```python
from build123d import *

# Parameters (mm, degrees)
SKETCH_1_W          = 2.91
SKETCH_1_H          = 12.7
EXTRUDE_1_DEPTH     = 3
EXTRUDE_2_DEPTH     = 3
CUT_EXTRUDE_3_DEPTH = 3
SKETCH_3_W          = 1.93
SKETCH_3_H          = 2.895
CUT_EXTRUDE_1_DEPTH = 3


with BuildPart() as part:
    # 스케치1 → 보스-돌출1 (new body)
    with BuildSketch(Plane(origin=(0, 0, 0), x_dir=(1, 0, 0), z_dir=(0, 1, 0))):
        Polygon((-17, -33.75), (-17, 33.75), (-4.66, 33.75), (-1.75, 33.75), (1.75, 33.75), (4.66, 33.75), (17, 33.75), (17, -33.75), (4.66, -33.75), (4.66, -19.81), (1.75, -19.81), (1.75, -33.75), (-1.75, -33.75), (-1.75, -19.81), (-4.66, -19.81), (-4.66, -33.75), align=None)
        with Locations((-3.205, 11.24)):
            Rectangle(SKETCH_1_W, SKETCH_1_H, mode=Mode.SUBTRACT)
        with Locations((-3.205, -7.46)):
            Rectangle(SKETCH_1_W, SKETCH_1_H, mode=Mode.SUBTRACT)
        with Locations((3.205, 11.24)):
            Rectangle(SKETCH_1_W, SKETCH_1_H, mode=Mode.SUBTRACT)
        with Locations((3.205, -7.46)):
            Rectangle(SKETCH_1_W, SKETCH_1_H, mode=Mode.SUBTRACT)
    extrude(amount=EXTRUDE_1_DEPTH)

    # 스케치2 → 보스-돌출2 (add)
    with BuildSketch(Plane(origin=(0, 3, 0), x_dir=(1, 0, 0), z_dir=(0, 1, 0))):
        with BuildLine():
            Line((-17, -33.75), (-17, 33.75))
            ThreePointArc((-17, 33.75), (-37.789714209, 0), (-17, -33.75))
        make_face()
        with BuildLine():
            ThreePointArc((-17, -33.75), (0, -37.789714209), (17, -33.75))
            Line((17, -33.75), (4.66, -33.75))
            Line((4.66, -33.75), (1.75, -33.75))
            Line((1.75, -33.75), (-1.75, -33.75))
            Line((-1.75, -33.75), (-4.66, -33.75))
            Line((-4.66, -33.75), (-17, -33.75))
        make_face()
        with BuildLine():
            ThreePointArc((37.789714209, 0), (32.175205062, 19.819653862), (17, 33.75))
            Line((17, 33.75), (17, -33.75))
            ThreePointArc((17, -33.75), (32.175205062, -19.819653862), (37.789714209, 0))
        make_face()
        with BuildLine():
            Line((-17, 33.75), (17, 33.75))
            ThreePointArc((17, 33.75), (0, 37.789714209), (-17, 33.75))
        make_face()
    extrude(amount=-EXTRUDE_2_DEPTH)

    # 스케치5 → 컷-돌출3 (cut)
    with BuildSketch(Plane(origin=(0, 3, 0), x_dir=(1, 0, 0), z_dir=(0, 1, 0))):
        with BuildLine():
            Line((-34.476203601, -4.66), (-31.537469067, -4.66))
            Line((-31.537469067, -4.66), (-31.537469067, 14.687146066))
            ThreePointArc((-31.537469067, 14.687146066), (-34.395192397, 5.224457362), (-34.476203601, -4.66))
        make_face()
        with BuildLine():
            Line((-24.537469067, 24.662457836), (-24.537469067, -4.66))
            Line((-24.537469067, -4.66), (-21.598734534, -4.66))
            Line((-21.598734534, -4.66), (-21.598734534, 27.273043125))
            ThreePointArc((-21.598734534, 27.273043125), (-23.10500183, 26.009288825), (-24.537469067, 24.662457836))
        make_face()
        with BuildLine():
            Line((-14.598734534, 31.578492123), (-14.598734534, -4.66))
            Line((-14.598734534, -4.66), (-11.66, -4.66))
            Line((-11.66, -4.66), (-11.66, 32.777562672))
            ThreePointArc((-11.66, 32.777562672), (-13.143048633, 32.211558288), (-14.598734534, 31.578492123))
        make_face()
        with BuildLine():
            Line((31.578492123, 14.598734534), (11.66, 14.598734534))
            Line((11.66, 14.598734534), (11.66, 11.66))
            Line((11.66, 11.66), (32.777562672, 11.66))
            ThreePointArc((32.777562672, 11.66), (32.211558288, 13.143048633), (31.578492123, 14.598734534))
        make_face()
        with BuildLine():
            Line((24.662457836, 24.537469067), (11.66, 24.537469067))
            Line((11.66, 24.537469067), (11.66, 21.598734534))
            Line((11.66, 21.598734534), (27.273043125, 21.598734534))
            ThreePointArc((27.273043125, 21.598734534), (26.009288825, 23.10500183), (24.662457836, 24.537469067))
        make_face()
        with BuildLine():
            Line((11.66, 31.537469067), (14.687146066, 31.537469067))
            ThreePointArc((14.687146066, 31.537469067), (13.188156979, 32.193116194), (11.66, 32.777562672))
            Line((11.66, 32.777562672), (11.66, 31.537469067))
        make_face()
        with BuildLine():
            Line((14.598734534, -31.578492123), (14.598734534, 4.66))
            Line((14.598734534, 4.66), (11.66, 4.66))
            Line((11.66, 4.66), (11.66, -32.777562672))
            ThreePointArc((11.66, -32.777562672), (13.143048633, -32.211558288), (14.598734534, -31.578492123))
        make_face()
        with BuildLine():
            Line((24.537469067, -24.662457836), (24.537469067, 4.66))
            Line((24.537469067, 4.66), (21.598734534, 4.66))
            Line((21.598734534, 4.66), (21.598734534, -27.273043125))
            ThreePointArc((21.598734534, -27.273043125), (23.10500183, -26.009288825), (24.537469067, -24.662457836))
        make_face()
        with BuildLine():
            Line((31.537469067, 4.66), (31.537469067, -14.687146066))
            ThreePointArc((31.537469067, -14.687146066), (34.395192397, -5.224457362), (34.476203601, 4.66))
            Line((34.476203601, 4.66), (31.537469067, 4.66))
        make_face()
        with BuildLine():
            Line((-31.578492123, -14.598734534), (-11.66, -14.598734534))
            Line((-11.66, -14.598734534), (-11.66, -11.66))
            Line((-11.66, -11.66), (-32.777562672, -11.66))
            ThreePointArc((-32.777562672, -11.66), (-32.211558288, -13.143048633), (-31.578492123, -14.598734534))
        make_face()
        with BuildLine():
            Line((-24.662457836, -24.537469067), (-11.66, -24.537469067))
            Line((-11.66, -24.537469067), (-11.66, -21.598734534))
            Line((-11.66, -21.598734534), (-27.273043125, -21.598734534))
            ThreePointArc((-27.273043125, -21.598734534), (-26.009288825, -23.10500183), (-24.662457836, -24.537469067))
        make_face()
        with BuildLine():
            Line((-11.66, -31.537469067), (-14.687146066, -31.537469067))
            ThreePointArc((-14.687146066, -31.537469067), (-13.188156979, -32.193116194), (-11.66, -32.777562672))
            Line((-11.66, -32.777562672), (-11.66, -31.537469067))
        make_face()
    extrude(amount=-CUT_EXTRUDE_3_DEPTH, mode=Mode.SUBTRACT)

    # 스케치3 → 컷-돌출1 (cut)
    with BuildSketch(Plane(origin=(0, 3, 0), x_dir=(1, 0, 0), z_dir=(0, 1, 0))):
        Polygon((-13.921720976, -29.640380671), (-16.485116171, -28.295007088), (-15.588200449, -26.586076958), (-13.024805254, -27.931450541), align=None)
        Polygon((-29.640380671, 13.921720976), (-28.295007088, 16.485116171), (-26.586076958, 15.588200449), (-27.931450541, 13.024805254), align=None)
        Polygon((13.921720976, 29.640380671), (16.485116171, 28.295007088), (15.588200449, 26.586076958), (13.024805254, 27.931450541), align=None)
        Polygon((26.876754365, 18.708462151), (28.424032932, 16.261636853), (26.792816067, 15.230117809), (25.2455375, 17.676943106), align=None)
        Polygon((29.640380671, -13.921720976), (28.295007088, -16.485116171), (26.586076958, -15.588200449), (27.931450541, -13.024805254), align=None)
        Polygon((-28.294726577, -6.082986865), (-27.545445441, -8.879342132), (-25.681208596, -8.379821375), (-26.430489732, -5.583466108), align=None)
        Polygon((-27.545445441, 8.879342132), (-28.294726577, 6.082986865), (-26.430489732, 5.583466108), (-25.681208596, 8.379821375), align=None)
        Polygon((27.545445441, -8.879342132), (28.294726577, -6.082986865), (26.430489732, -5.583466108), (25.681208596, -8.379821375), align=None)
        Polygon((-18.947986862, -16.900912731), (-16.900912731, -18.947986862), (-15.536196643, -17.583270774), (-17.583270774, -15.536196643), align=None)
        Polygon((-16.900912731, 18.947986862), (-18.947986862, 16.900912731), (-17.583270774, 15.536196643), (-15.536196643, 17.583270774), align=None)
        with BuildLine():
            Line((15.862041837, -7.0175654), (18.772041837, -7.0175654))
            Line((18.772041837, -7.0175654), (18.772041837, -4.1605654))
            Line((18.772041837, -4.1605654), (19.614041677, -4.1605654))
            ThreePointArc((19.614041677, -4.1605654), (19.916683492, -4.035207055), (20.042041837, -3.73256524))
            Line((20.042041837, -3.73256524), (20.042041837, -2.30256556))
            ThreePointArc((20.042041837, -2.30256556), (19.916683492, -1.999923745), (19.614041677, -1.8745654))
            Line((19.614041677, -1.8745654), (18.772041837, -1.8745654))
            Line((18.772041837, -1.8745654), (18.772041837, 0.9824346))
            Line((18.772041837, 0.9824346), (15.862041837, 0.9824346))
            Line((15.862041837, 0.9824346), (15.862041837, -7.0175654))
        make_face()
        Polygon((18.708462151, -26.876754365), (16.261636853, -28.424032932), (15.230117809, -26.792816067), (17.676943106, -25.2455375), align=None)
        Polygon((16.900912731, -18.947986862), (18.947986862, -16.900912731), (17.583270774, -15.536196643), (15.536196643, -17.583270774), align=None)
        Polygon((-10.527707159, 15.339523687), (-8.020563615, 16.787023687), (-7.055563615, 15.115594658), (-9.562707159, 13.668094658), align=None)
        with Locations((-17.583270774, 0)):
            Rectangle(SKETCH_3_W, SKETCH_3_H)
        Polygon((8.020563615, 16.787023687), (10.527707159, 15.339523687), (9.562707159, 13.668094658), (7.055563615, 15.115594658), align=None)
        Polygon((10.527707159, -15.339523687), (8.020563615, -16.787023687), (7.055563615, -15.115594658), (9.562707159, -13.668094658), align=None)
        Polygon((-8.020563615, -16.787023687), (-10.527707159, -15.339523687), (-9.562707159, -13.668094658), (-7.055563615, -15.115594658), align=None)
    extrude(amount=-CUT_EXTRUDE_1_DEPTH, mode=Mode.SUBTRACT)


solid = part.part
```
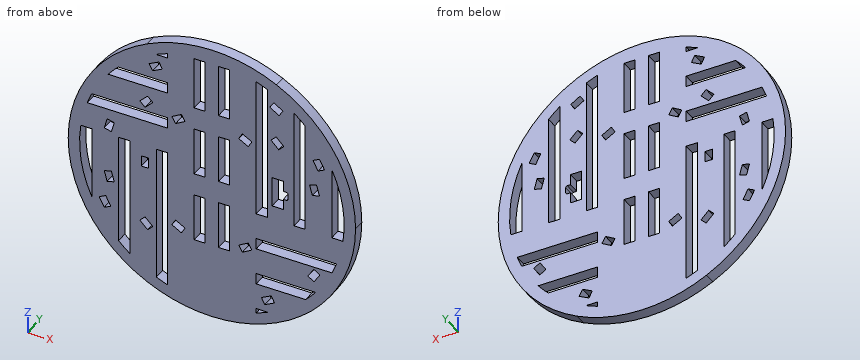
Read the model definition and answer for the solid it produces. Units are mm, in the model's axes. Give positions to 0.01 mm unless a question says otherwise; leave off trailing zeros. Loops run counter-clockwise (first coordinate to the right, second up) from the corner with the lowest first, then second, coordinate; pieces in that order, holes last.
Item 1: The part is cut by section B-B (x = 30.5). Write down the section's boundary in (y, z), and give its area (3 significant figures).
Item 2: Each of these flat-tipped pins is pushed along its axis until it touches: pin 1 Ø0.9 at (x, y) = (17.5, 1.5) entering from -Z; pin 2 Ø1.5 at (x, y) = (2.5, 2) entering from +Z; pin 3 Ø1.5 at (x, y) = (-6.5, 2) entering from -Z. Where does it stop, or does it pass through?
Item 3: Find the intervals of material crossed by line 1 along Z through (x, y) = (-19, 2.1); line 2 along X through (y, z) = (0.55, -24.5); line 3 along X through (y, z) = (1.1, 22), in increasing order.
Item 4: The part is cut by section A-A (z = -3.5). Write down the section's boundary in (x, y).
Item 5: The part is cut by section C-C (y = 1.45). Give the number of separate pieces and of enclosed holes in the cut face, and give its area (3 significant figures).
Taken from the geometry:
1. outline: (0, -22.31) - (3, -22.31) - (3, -14.6) - (0, -14.6) - close; (0, -11.66) - (3, -11.66) - (3, 22.31) - (0, 22.31) - close
1. area: 125 mm2
2. pin 1: stops at z = -33.72
2. pin 2: stops at z = 37.75
2. pin 3: stops at z = -37.35
3. line 1: z = -32.67 to 11.66, 14.6 to 21.6, 24.54 to 32.67
3. line 2: x = -28.77 to -24.54, -21.6 to -14.6, -11.66 to 11.66, 24.7 to 28.77
3. line 3: x = -30.73 to -26.95, -11.66 to -4.66, -1.75 to 1.75, 4.66 to 11.66, 14.6 to 21.6, 24.54 to 30.73
4. outline: (-37.63, 0) - (-34.61, 0) - (-34.61, 3) - (-37.63, 3) - close; (-31.54, 0) - (-24.54, 0) - (-24.54, 3) - (-31.54, 3) - close; (-21.6, 0) - (-14.6, 0) - (-14.6, 3) - (-21.6, 3) - close; (-11.66, 0) - (11.66, 0) - (11.66, 3) - (-11.66, 3) - close; (14.6, 0) - (21.6, 0) - (21.6, 3) - (14.6, 3) - close; (24.54, 0) - (31.54, 0) - (31.54, 3) - (24.54, 3) - close; (34.61, 0) - (37.63, 0) - (37.63, 3) - (34.61, 3) - close
5. separate pieces: 1
5. enclosed holes: 36
5. area: 3,440 mm2
